Geometry: see drawing. Coordinates: mm, zero at the bounding-box minimum. Give positions to 0.01 mm unless a question says otherwise; leave off trailing zeros. Write each loop counter-clockwise with the first axis right and the second up, starting at its lowest first coordinate (ties: lowest second). Pieces come first, ordered by that corner, then holes.
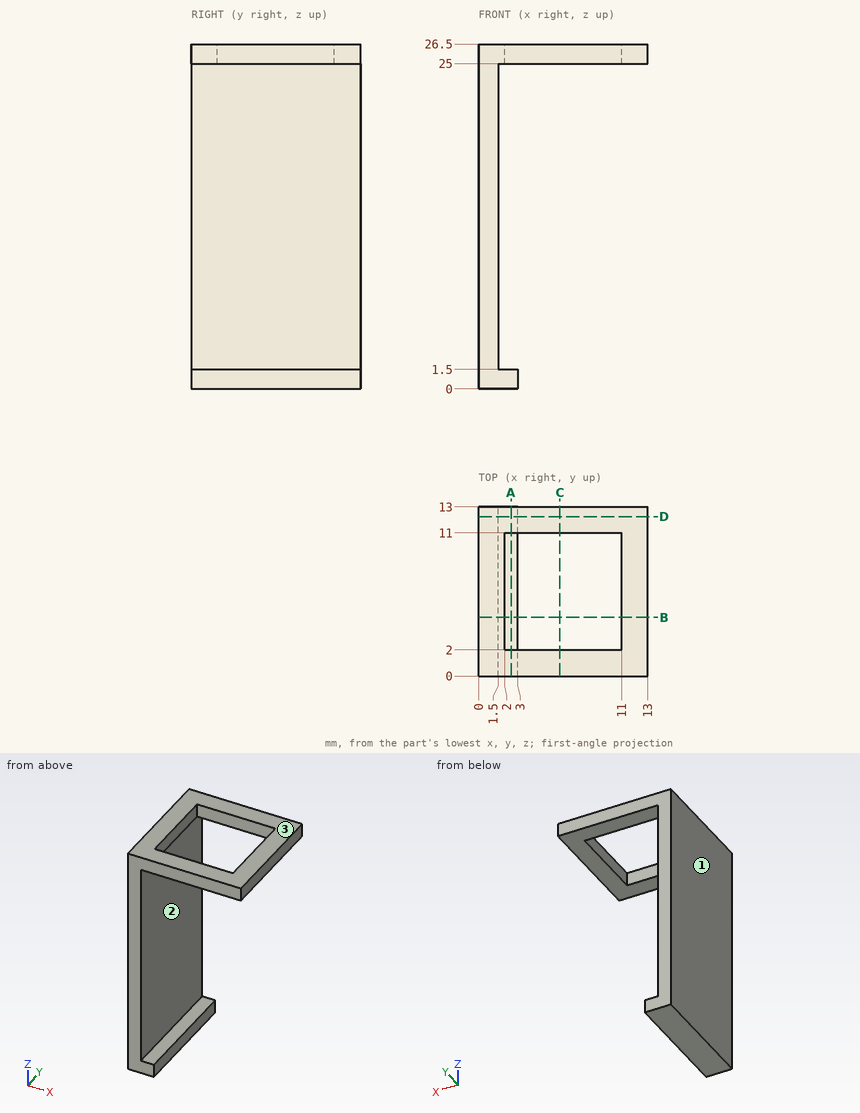
Q1. Section C-C, the plane x = 6.25. Return the cut outline in (y, z), then the cut area to 3 significant figures.
Q2. Section D-D, the plane y = 12.25. Return the cut outline in (x, z), then the cut area to 4 significant figures.
Q3. Mould query, pull axis Z, two halves, no side actions, for the marked faces 1, 2 and 3. Classes: +Z half, -Z half, draft (parallel to the pull), parting line (faces both ways), or undercut.
Q4. Material intervals for line 1 along X through (y, z) = (6, 25.25); line 2 along Z through (x, y) = (12.25, 5); line 3 along X through (y, z) = (6.5, 21.5), sorted ascending.
Q5. Section A-A, the plane x = 2.5. Return the cut outline in (y, z), then the cut area to 3 significant figures.
Q6. Section B-B, the plane y = 4.5. Return the cut outline in (x, z).
Q7. Pin query (flat end, axial travel): pin 1 (0.8 mm diameter, centred on x = 2.5, y = 9, fed in from +Z); pin 2 (4 mm diameter, centred on y = 8, z = 11, fed in from +X); pin 3 (1.6 mm diameter, centred on y = 4, z = 0.5, fed in from +X). Return the tip coordinate at first contact, or that it passes through.
Solutions:
1. outline: (0, 25) - (2, 25) - (2, 26.5) - (0, 26.5) - close; (11, 25) - (13, 25) - (13, 26.5) - (11, 26.5) - close
1. area: 6.00 mm2
2. outline: (0, 0) - (3, 0) - (3, 1.5) - (1.5, 1.5) - (1.5, 25) - (13, 25) - (13, 26.5) - (0, 26.5) - close
2. area: 59.25 mm2
3. face 1: draft
3. face 2: undercut
3. face 3: +Z half
4. line 1: x = 0 to 2, 11 to 13
4. line 2: z = 25 to 26.5
4. line 3: x = 0 to 1.5
5. outline: (0, 0) - (13, 0) - (13, 1.5) - (0, 1.5) - close; (0, 25) - (2, 25) - (2, 26.5) - (0, 26.5) - close; (11, 25) - (13, 25) - (13, 26.5) - (11, 26.5) - close
5. area: 25.5 mm2
6. outline: (0, 0) - (3, 0) - (3, 1.5) - (1.5, 1.5) - (1.5, 25) - (2, 25) - (2, 26.5) - (0, 26.5) - close; (11, 25) - (13, 25) - (13, 26.5) - (11, 26.5) - close
7. pin 1: stops at z = 1.5
7. pin 2: stops at x = 1.5
7. pin 3: stops at x = 3
